Verification items for the finished model (mm, model axes). A direction names the side the tool comes from. Round coordinates to 2 decimals unless told otherwise and drop trailing zeros. Write each loop counter-clockwise with the first axis right and the second up, starting at its lowest first coordinate (ties: lowest second). Pieces come first, ordered by that corner, then holes. Notation, with made-up numbers: (4.5, 2) - (14.5, 2) arc R24 ccw to (14.5, 30) - close; hole circle Ø3 at (62, 62.5). An arc over 180 degrees is marked (long way). Answer as a JSON object with one key per item and string values.
```python
from build123d import *

# Parameters (mm, degrees)
SKETCH1_W           = 27
SKETCH1_H           = 20
SKETCH1_R           = 1.5
SKETCH1_W_2         = 18.8
SKETCH1_H_2         = 13.5
BOSS_EXTRUDE1_DEPTH = 4
SKETCH2_R           = 1.5
CUT_EXTRUDE2_DEPTH  = 6
CUT_EXTRUDE3_START  = -6
SKETCH5_R           = 1.5
CUT_EXTRUDE3_DEPTH  = 6


with BuildPart() as part:
    # Sketch1 → Boss-Extrude1 (new body)
    with BuildSketch(Plane(origin=(0, 0, 0), x_dir=(1, 0, 0), z_dir=(0, 1, 0))):
        with Locations((0, 1.25)):
            Rectangle(SKETCH1_W, SKETCH1_H)
        with Locations(Location((-7.5, 8.75, 0), (0, 0, 270))):
            Circle(SKETCH1_R, mode=Mode.SUBTRACT)
        with Locations(Location((7.5, 8.75, 0), (0, 0, 90))):
            Circle(SKETCH1_R, mode=Mode.SUBTRACT)
        Rectangle(SKETCH1_W_2, SKETCH1_H_2, mode=Mode.SUBTRACT)
    extrude(amount=BOSS_EXTRUDE1_DEPTH)

    # Sketch2 → Cut-Extrude2 (cut)
    with BuildSketch(Plane(origin=(0, 0, -11.25), x_dir=(-1, 0, 0), z_dir=(0, 0, -1))):
        with Locations((11, 2)):
            Circle(SKETCH2_R)
        with Locations((-11, 2)):
            Circle(SKETCH2_R)
    extrude(amount=-CUT_EXTRUDE2_DEPTH, mode=Mode.SUBTRACT)

    # Sketch5 → Cut-Extrude3 (cut)
    with BuildSketch(Plane.XY.offset(8.75).offset(CUT_EXTRUDE3_START)):
        with Locations(Location((11, 2, 0), (0, 0, 180))):
            Circle(SKETCH5_R)
        with Locations(Location((-11, 2, 0), (0, 0, 180))):
            Circle(SKETCH5_R)
    extrude(amount=CUT_EXTRUDE3_DEPTH, mode=Mode.SUBTRACT)


solid = part.part
```
1. Cross-section at C-C (y = 2). Record the boundary of the cut face in (x, z).
Completed:
{"outline": "(-13.5, -11.25) - (-12.5, -11.25) - (-12.5, -5.25) - (-9.5, -5.25) - (-9.5, -11.25) - (9.5, -11.25) - (9.5, -5.25) - (12.5, -5.25) - (12.5, -11.25) - (13.5, -11.25) - (13.5, 8.75) - (12.5, 8.75) - (12.5, 2.75) - (9.5, 2.75) - (9.5, 8.75) - (-9.5, 8.75) - (-9.5, 2.75) - (-12.5, 2.75) - (-12.5, 8.75) - (-13.5, 8.75) - close; hole (-9.4, -6.75) - (9.4, -6.75) - (9.4, 6.75) - (-9.4, 6.75) - close; hole circle Ø3 at (-7.5, -8.75); hole circle Ø3 at (7.5, -8.75)"}
2. Cross-section at B-B (x = -7.5). Record the boundary of the cut face in (y, z).
Completed:
{"outline": "(0, -11.25) - (4, -11.25) - (4, -10.25) - (0, -10.25) - close; (0, -7.25) - (4, -7.25) - (4, -6.75) - (0, -6.75) - close; (0, 6.75) - (4, 6.75) - (4, 8.75) - (0, 8.75) - close"}
3. Go/stop test with flat-tipped pins: pin 1 (1.5 mm diameter, centred on x = -11.5, y = 1.5, fed in from +Z); pin 2 (0.9 mm diameter, centred on x = 10.5, y = 2, fed in from -Z); pin 3 (5 mm diameter, centred on x = 7.5, z = -8.75, fed in from -Y). Record where each tip stops, or that it passes through.
Completed:
{"pin 1": "stops at z = 2.75", "pin 2": "stops at z = -5.25", "pin 3": "stops at y = 0"}
4. Access from +Z, -Z, +X, -X, +Y, -Y to the whole of each face (thin tool, end or side, straight path). Record for faces 4 (the face through (-9.4, 2, 0)), 5 (the face through (-11, 2, 2.75)), 6 (the face through (-11, 2, -5.25)).
Completed:
{"face 4": "+Y, -Y", "face 5": "+Z", "face 6": "-Z"}
5. Material ranges on probe 1 along X at (y, z) = (2, 7.3); probe 2 along X at (y, z) = (3.85, -1.5); probe 3 along Z at (x, y) = (-1.25, 0.3), recorded low to high. Write a range as from..to.
Completed:
{"probe 1": "x = -13.5..-12.5, -9.5..9.5, 12.5..13.5", "probe 2": "x = -13.5..-9.4, 9.4..13.5", "probe 3": "z = -11.25..-6.75, 6.75..8.75"}
6. Cross-section at D-D (z = 1). Record the boundary of the cut face in (x, y), plus the area to 3 significant figures.
Completed:
{"outline": "(-13.5, 0) - (-9.4, 0) - (-9.4, 4) - (-13.5, 4) - close; (9.4, 0) - (13.5, 0) - (13.5, 4) - (9.4, 4) - close", "area": "32.8 mm^2"}
7. Mould release check, pull along Z, two halves, no side actions. Record for faces 1 (the face through (11, 2, -5.25)), 2 (the face through (12.5, 2.07, -8.29)), 3 (the face through (-8.964, 1.972, -9.075)): released by +Z, released by -Z, zero draft, split by the parting line, or undercut.
Completed:
{"face 1": "released by -Z", "face 2": "zero draft", "face 3": "undercut"}
8. Cross-section at A-A (z = -8.75). Record the boundary of the cut face in (x, y), plus the area to 3 significant figures.
Completed:
{"outline": "(-13.5, 0) - (-9, 0) - (-9, 4) - (-13.5, 4) - close; (-6, 0) - (6, 0) - (6, 4) - (-6, 4) - close; (9, 0) - (13.5, 0) - (13.5, 4) - (9, 4) - close; hole circle Ø3 at (-11, 2); hole circle Ø3 at (11, 2)", "area": "69.9 mm^2"}
